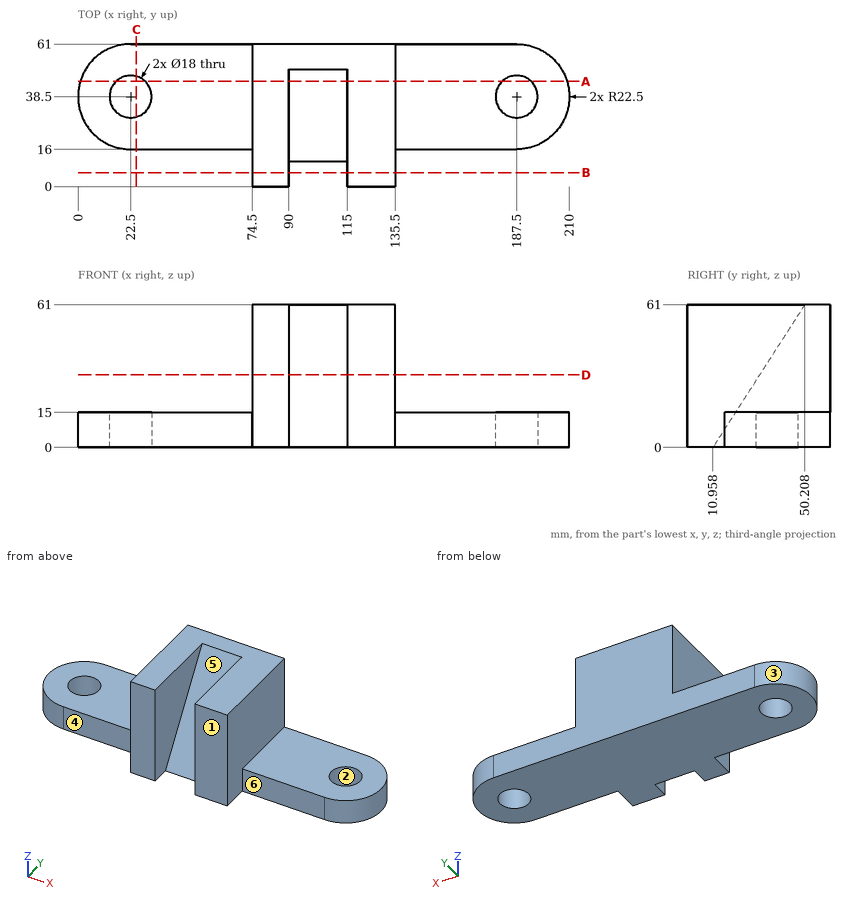
Study the drawing (mm; zero at the part's minimum x, y, z) and answer. A direction names the side the tool comes from. Round coordinates to 2 decimals unless told otherwise and drop trailing zeros. Write each loop counter-clockwise with the first axis right and the second up, starting at its lowest first coordinate (ties: lowest second). Pieces come first, ordered by that corner, then holes. Notation, with made-up numbers: (71.25, 44) -> (92.25, 44) arc R22 ccw to (92.25, 51) -> close; hole circle Ø11 at (76, -6.5). An arc over 180 degrees is marked (long way). Write item = value, one per line.
1) Section A-A on y = 45 is taken. Write down the section's boundary in (x, z) (1 decimal).
Check values:
outline = (1, 0) -> (16.3, 0) -> (16.3, 15) -> (1, 15) -> close; (28.7, 0) -> (181.3, 0) -> (181.3, 15) -> (135.5, 15) -> (135.5, 61) -> (115, 61) -> (115, 52.9) -> (90, 52.9) -> (90, 61) -> (74.5, 61) -> (74.5, 15) -> (28.7, 15) -> close; (193.7, 0) -> (209, 0) -> (209, 15) -> (193.7, 15) -> close
2) Section D-D on z = 31 is taken. Write down the section's boundary in (x, y) (1 decimal), plus the area to 3 significant figures.
Check values:
outline = (74.5, 0) -> (90, 0) -> (90, 30.9) -> (115, 30.9) -> (115, 0) -> (135.5, 0) -> (135.5, 61) -> (74.5, 61) -> close
area = 2,950 mm²
3) Section B-B on y = 6 is taken. Write down the section's boundary in (x, z), plus the area to 3 significant figures.
Check values:
outline = (74.5, 0) -> (90, 0) -> (90, 61) -> (74.5, 61) -> close; (115, 0) -> (135.5, 0) -> (135.5, 61) -> (115, 61) -> close
area = 2,200 mm²
4) Section C-C on x = 25 is taken. Write down the section's boundary in (y, z).
Check values:
outline = (16, 0) -> (29.85, 0) -> (29.85, 15) -> (16, 15) -> close; (47.15, 0) -> (61, 0) -> (61, 15) -> (47.15, 15) -> close
5) Which of the six approach directions +Z, -Z, +X, -X, +Y, -Y give full straight-line access (tool end or side, diameter ignored) to the marked faces 4, 5 and 6?
Check values:
face_4 = +Z, -Z, -X, -Y
face_5 = +Z, -Y
face_6 = +Z, -Z, +X, -Y
6) For a pull along X with two mould halves and no side action, classify the marked faces 1, 2 and 3 as released by +X, released by -X, zero draft, split by the parting line, or undercut.
Check values:
face_1 = zero draft
face_2 = undercut
face_3 = released by -X
7) Given pin 1 (16.5 mm diameter, centred on x = 49, z = 6.5, fed in from -Y); pin 2 (6 mm diameter, centred on y = 26.5, z = 25.5, fed in from +X); pin 3 (4 mm diameter, centred on y = 22.5, z = 29, fed in from -X), each flat-ended and moving along its own axis, determine where each tip first touches the part or whether it passes through.
Check values:
pin_1 = 16
pin_2 = 135.5
pin_3 = 74.5
8) Straight lines are drawn through the part: line 1 along Y through (x, z) = (22, 3) (1 decimal); line 2 along X through (y, z) = (3.5, 10); line 3 along Z through (x, y) = (199, 29.5). For each, find the intervals that lie inside material, in ascending order. Write a range as [from, to].
Check values:
line_1 = [16, 29.5], [47.5, 61]
line_2 = [74.5, 90], [115, 135.5]
line_3 = [0, 15]
